CAD build for the part. Positions are in the model's coordinates, mm. A direction names the side the tool comes from. Give positions to 0.01 mm unless a question says otherwise; leave off trailing zeros. Write each loop counter-clockwise with the first axis right and the second up, starting at its lowest first coordinate (ties: lowest second). Pieces come first, ordered by that corner, then holes. Notation, with made-up numbers: (-31.5, 77) - (26.5, 77) arc R26 cw to (26.5, 114) - close; hole circle Ø11 at (41, -35.5). An arc over 180 degrees is marked (long way). Put each result on its own line as item: value. Start each with the question number.
1. Cut at D-D on x = -20. List the corners of the cut face in (y, z).
2. Tool access for faces 5 (the flat face through (16, 3, 11)), 6 (the flat face through (-20, 8, -14)), 7 (the flat face through (-16, 3, -11)), 8 (the cylindrical face through (-20, 4, 8)), 9 (the cylindrical face through (-5.96, 7.6, 1.88)): list every direction of +Z, -Z, +X, -X, +Y, -Y with a clear straight run to the whole face (end or side of a thin tool).
3. Wall check: line 1 (X direction, y = 8, z = 0); line 2 (Z direction, x = 0, y = 3); line 3 (Z direction, x = 18.5, y = 17.75). Give the ranges that are in metal, low to high.
4. Mould opens along Z. For faces 1 (the flat face through (20, 4, -16)), 2 (the flat face through (-20, 4, 16)), 3 (the cylindrical face through (20, 4, 8)), 4 (the flat face through (-24, 4, 0)) say: +Z half, -Z half, draft (parallel to the pull), parting line (faces both ways), or undercut.
5. Drop flat-ended pins along their axis: pin 1 (2.5 mm diameter, centred on x = 12.5, z = 2, fed in from +Y); pin 2 (4.5 mm diameter, centred on x = 15, y = 13.5, fed in from -Z); pin 3 (3 mm diameter, centred on x = -19, z = -13, fed in from +Y). Give the stop position or say it passes through.
6. Cut at C-C on y = 5.75. Give the number of separate pieces and of enclosed holes in the cut face, and give its area (3 significant figures).
7. Cut at B-B on z = -8. List the corners of the cut face in (x, y).
8. Cut at A-A on z = -13. List the corners of the cut face in (x, y), and give its area (3 significant figures).
from build123d import *

# Parameters (mm, degrees)
SKETCH1_R                = 10
PEN_CAP_DEPTH            = 25
SKETCH2_W                = 48
SKETCH2_H                = 8
HOOK_STRUCTURE_DEPTH     = 20
PEN_CENTERING_HOLE_D     = 12.5
PEN_CENTERING_HOLE_DEPTH = 15
PEN_CENTERING_HOLE_TIP   = 6.25
HOOKS_DEPTH              = 8
CORNER_DEC_R             = 10


with BuildPart() as part:
    # Sketch1 → Pen Cap (new body)
    with BuildSketch(Plane(origin=(0, 0, 0), x_dir=(1, 0, 0), z_dir=(0, 1, 0))):
        Circle(SKETCH1_R)
    extrude(amount=PEN_CAP_DEPTH)

    # Sketch2 → Hook Structure (add)
    with BuildSketch(Plane.XZ):
        Rectangle(SKETCH2_W, SKETCH2_H)
    extrude(amount=-HOOK_STRUCTURE_DEPTH)

    # Pen Centering Hole
    with Locations(Plane.XZ):
        with Locations((0, 0)):
            Hole(PEN_CENTERING_HOLE_D / 2, depth=PEN_CENTERING_HOLE_DEPTH)
            with Locations((0, 0, -(PEN_CENTERING_HOLE_DEPTH + PEN_CENTERING_HOLE_TIP / 2))):  # 90° drill point
                Cone(0, PEN_CENTERING_HOLE_D / 2, PEN_CENTERING_HOLE_TIP, mode=Mode.SUBTRACT)

    # Sketch6 → Hooks (add)
    with BuildSketch(Plane(origin=(24, 0, 0), x_dir=(0, 0, -1), z_dir=(1, 0, 0))):
        with BuildLine():
            Line((-4, 0), (-16, 0))
            Line((-16, 0), (-16, 8))
            Line((-16, 8), (-12, 8))
            ThreePointArc((-12, 8), (-8, 4), (-4, 8))
            Line((-4, 8), (-4, 0))
        make_face()
        with BuildLine():
            Line((4, 8), (4, 0))
            Line((4, 0), (16, 0))
            Line((16, 0), (16, 8))
            Line((16, 8), (12, 8))
            ThreePointArc((12, 8), (8, 4), (4, 8))
        make_face()
    hooks = extrude(amount=-HOOKS_DEPTH)

    # Hook Mirror: Hooks across plane
    add(hooks.mirror(Plane(origin=(0, 0, 0), x_dir=(0, 0, 1), z_dir=(1, 0, 0))))

    # Corner Dec
    corner_dec_edges = [part.edges().sort_by_distance(p)[0] for p in [
        (-24, 20, 0),
        (24, 20, 0),
    ]]
    fillet(corner_dec_edges, radius=CORNER_DEC_R)


solid = part.part
Report:
1. outline: (0, -16) - (8, -16) - (8, -12) arc R4 cw to (8, -4) - (18, -4) - (18, 4) - (8, 4) arc R4 cw to (8, 12) - (8, 16) - (0, 16) - close
2. face 5: +Z, +Y, -Y
2. face 6: -Z, +X, -X, +Y
2. face 7: -Z, +Y, -Y
2. face 8: -X, +Y
2. face 9: -Y
3. line 1: x = -24 to -6.25, 6.25 to 24
3. line 2: z = -10 to -6.25, 6.25 to 10
3. line 3: z = -4 to 4
4. face 1: -Z half
4. face 2: +Z half
4. face 3: undercut
4. face 4: draft
5. pin 1: stops at y = 20
5. pin 2: stops at z = -4
5. pin 3: stops at y = 8
6. separate pieces: 5
6. enclosed holes: 1
6. area: 592 mm²
7. outline: (-24, 0) - (-16, 0) - (-16, 4) - (-24, 4) - close; (-6, 0) - (6, 0) - (6, 25) - (-6, 25) - close; (16, 0) - (24, 0) - (24, 4) - (16, 4) - close
8. outline: (-24, 0) - (-16, 0) - (-16, 8) - (-24, 8) - close; (16, 0) - (24, 0) - (24, 8) - (16, 8) - close
8. area: 128 mm²
